The model under review builds one solid part; all positions refer to its coordinate system, in mm. A direction names the side the tool comes from. Give positions to 0.01 mm unless a question says otherwise; leave off trailing zeros. Write each loop counter-clockwise with the first axis right and the second up, starting at its lowest first coordinate (ties: lowest second). Pieces come first, ordered by that corner, then holes.
Autodesk Inventor part; units mm, degrees
ref_plane "YZ Plane" through (0, 0, 0) normal (1, 0, 0) x (0, 1, 0)
ref_plane "XZ Plane" through (0, 0, 0) normal (0, 1, 0) x (-1, 0, 0)
ref_plane "XY Plane" through (0, 0, 0) normal (0, 0, 1) x (1, 0, 0)
sketch "Sketch1" plane through (0, 0, 0) normal (0, 0, 1) x (1, 0, 0)
  line L0 (0, 0) -> (29, 0)
  line L1 (29, 0) -> (29, -162)
  line L2 (29, -162) -> (0, -162)
  line L3 (0, -162) -> (0, 0) construction
  line L4 (0, 0) -> (-29, 0)
  line L5 (-29, 0) -> (-29, -162)
  line L6 (-29, -162) -> (0, -162)
  dimension "d0" = 29
  dimension "d1" = 162
extrude "Extrusion1" add sketch "Sketch1" along normal mid plane 67
sketch "Sketch3" plane through (0, 0, 0) normal (1, 0, 0) x (0, 1, 0)
  line L0 (-162, 28.5) -> (-165, 28.5)
  line L1 (-165, 28.5) -> (-175.6066, 39.1066)
  line L2 (-162, 33.5) -> (0, 33.5)
  line L3 (-162, 33.5) -> (-162, -33.5)
  line L4 (-162, -28.5) -> (-190.0244, -28.5)
  line L5 (-190.0244, -28.5) -> (-216.6188, -1.9056)
  line L6 (-177.0208, 37.6924) -> (-169.2426, 29.9142)
  line L7 (-169.2426, 29.9142) -> (-207.4264, -8.2696)
  line L8 (-207.4264, -8.2696) -> (-215.2046, -0.4914)
  line L9 (-175.6066, 39.1066) -> (-177.0208, 37.6924)
  line L10 (-215.2046, -0.4914) -> (-216.6188, -1.9056)
  line L11 (0, -33.5) -> (-162, -33.5) construction
  point P0 (0, 0)
  dimension "d6" = 5
  dimension "d7" = 3
  dimension "d8" = 45
  dimension "d9" = 15
  dimension "d11" = 11
  dimension "d13" = 2
  dimension "d14" = 54
  dimension "d15" = 5
  dimension "d16" = 90
extrude "Extrusion2" add sketch "Sketch3" along normal mid plane 54
sketch "Sketch5" plane through (0, 0, 0) normal (1, 0, 0) x (0, 1, 0)
  line L0 (-207.4264, 68.098) -> (-169.2426, 29.9142)
  line L1 (-169.2426, 29.9142) -> (-207.4264, -8.2696)
  line L2 (-207.4264, -8.2696) -> (-245.6102, 29.9142)
  line L3 (-245.6102, 29.9142) -> (-207.4264, 68.098)
  line L4 (-169.2426, 29.9142) -> (-207.4264, -8.2696)
  line L5 (-177.0208, 37.6924) -> (-169.2426, 29.9142)
  line L6 (-207.4264, -8.2696) -> (-215.2046, -0.4914)
  point P0 (0, 0)
extrude "Extrusion3" add sketch "Sketch5" along normal mid plane 114
sketch "Sketch6" plane through (-29, 0, 33.5) normal (0, 1, 0) x (1, 0, 0)
  circle A0 centre (29, 33.5) radius 10
  dimension "d21" = 20
extrude "Extrusion4" cut sketch "Sketch6" against normal blind 10
sketch "Sketch7" plane through (57, 0, 0) normal (1, 0, 0) x (0, 0, -1)
  line L0 (-29.9142, -169.2426) -> (-68.098, -207.4264)
  line L1 (-68.098, -207.4264) -> (-29.9142, -245.6102)
  line L2 (-29.9142, -245.6102) -> (8.2696, -207.4264)
  line L3 (8.2696, -207.4264) -> (-29.9142, -169.2426)
  line L4 (-29.9142, -245.6102) -> (-29.9142, -169.2426) construction
  circle A0 centre (-29.9142, -207.4264) radius 27
  point P0 (0, 0)
extrude "Extrusion5" cut sketch "Sketch7" against normal blind 30 contours L3 A0 L0 | A0 L1 L0 | L3 L2 A0 | A0 L2 L1
move or copy body "Move Body1" bodies to move or copy 1 copy no rotation origin (0, 0, 0) rotation axis (1, 0, 0) rotation angle 90
move or copy body "Move Body2" bodies to move or copy 1 copy no rotation origin (0, 0, 0) rotation axis (0, 0, 1) rotation angle 90
move or copy body "Move Body3" bodies to move or copy 1 copy no translate (0, 0, -39)
properties part number "Sholder_Yaw"
1) Consider section D-D, the plane x = 43. Give the boundary of the cut face in (y, z), then the cut area to 3 significant figures.
2) Tool access review of faces 4 (the cylindrical face through (49.83, 42.21, -264.66)), 5 (the flat face through (0, 29, -119)), 6 (the cylindrical face through (9.76, -2.17, -43.93)), 7 (the flat face through (0, -29, -119)): name each direction out of +Z, -Z, +X, -X, +Y, -Y from which nothing blocks a thin tool from reaching the whole face with its end or side.
3) To check wall thickness, follow probe 1 along Y at (x, z) = (0, -44); probe 2 along X at (y, z) = (0, -47); probe 3 along X at (y, z) = (-17, -150.5). State the ranges of each line that lie inside material, in increasing order.
4) Consider section A-A, the plane y = 19.5. Give the boundary of the cut face in (x, z), then the cut area to 3 significant figures.
5) Consider section C-C, the plane x = -25.5. Give the boundary of the cut face in (y, z).
6) The part is to be moulded in two halves that separate along Z. For faces 1 (the flat face through (33.7, -0.4, -209.2)), 2 (the flat face through (30, -57, -247)), 3 (the flat face through (0, 0, -49)), say which applies: +Z half, -Z half, draft (parallel to the pull), parting line (faces both ways), or undercut.
7) Consider section B-B, the plane z = -235. Give the boundary of the cut face in (x, y).
8) Insertion check: pin 1 (2 mm diameter, centred on x = 29.5, z = -199, fed in from +Y); pin 2 (14 mm diameter, centred on y = -2.5, z = -213.5, fed in from -X); pin 3 (0.9 mm diameter, centred on y = 10, z = -203, fed in from +X). Each pin has a flat end and moves straight along its axis. Give the tip position at first contact, or say it passes through.
Answer block:
1. outline: (-57, -271.52) - (27, -271.52) - (27, -270.04) - (57, -270.04) - (57, -222.81) - (27, -222.81) - (27, -221.33) - (-57, -221.33) - close
1. area: 5,630 mm2
2. face 4: +Y
2. face 5: +Z, +X, -X, +Y
2. face 6: +Z
2. face 7: +Z, +X, -X, -Y
3. probe 1: y = -29 to -10, 10 to 29
3. probe 2: x = -33.5 to -10, 10 to 33.5
3. probe 3: x = -33.5 to 33.5
4. outline: (-33.5, -201) - (-28.5, -201) - (-28.5, -229.02) - (-1.91, -255.62) - (-0.49, -254.2) - (29.91, -284.61) - (68.1, -246.43) - (37.69, -216.02) - (39.11, -214.61) - (28.5, -204) - (28.5, -201) - (33.5, -201) - (33.5, -39) - (-33.5, -39) - close
4. area: 15,600 mm2
5. outline: (-29, -201) - (-27, -201) - (-27, -232.02) - (27, -232.02) - (27, -201) - (29, -201) - (29, -39) - (-29, -39) - close
6. face 1: undercut
6. face 2: draft
6. face 3: +Z half
7. outline: (-22.52, -27) - (3.16, -27) - (3.16, -57) - (56.67, -57) - (56.67, 27) - (54.38, 27) - (54.38, 57) - (5.45, 57) - (5.45, 27) - (-22.52, 27) - close
8. pin 1: stops at y = 29
8. pin 2: stops at x = -28.5
8. pin 3: stops at x = 28.5
